from build123d import *

# Parameters (mm, degrees)
SKETCH1_R           = 3.325
SKETCH1_R_2         = 8.5
BOSS_EXTRUDE1_DEPTH = 2.5


with BuildPart() as part:
    # Sketch1 → Boss-Extrude1 (new, symmetric)
    with BuildSketch(Plane.XY):
        with BuildLine():
            ThreePointArc((60.622067271, 14.206532436), (59.125498335, 14.810906809), (57.524692071, 15.016834632))
            Line((57.524692071, 15.016834632), (56.997116089, 14.994793348))
            Line((56.997116089, 14.994793348), (37.942484943, 14.198721238))
            ThreePointArc((37.942484943, 14.198721238), (29.810784304, 16.198484397), (24.018273447, 22.245833067))
            ThreePointArc((24.018273447, 22.245833067), (11.4864831, 29.488233713), (-0.397539124, 21.225779345))
            ThreePointArc((-0.397539124, 21.225779345), (-5.665447564, 14.71634399), (-13.602008261, 12.045274491))
            Line((-13.602008261, 12.045274491), (-32.656639407, 11.249202381))
            ThreePointArc((-32.656639407, 11.249202381), (-35.431571333, 10.60798438), (-37.643867273, 8.81434161))
            ThreePointArc((-37.643867273, 8.81434161), (-38.932803958, 4.139738531), (-36.53293032, -0.073796594))
            Line((-36.53293032, -0.073796594), (10.980057512, -36.923376572))
            ThreePointArc((10.980057512, -36.923376572), (14.305396611, -37.984745832), (17.530617501, -36.649704619))
            Line((17.530617501, -36.649704619), (61.804364137, 4.034578786))
            ThreePointArc((61.804364137, 4.034578786), (63.807395856, 9.422079897), (60.622067271, 14.206532436))
        make_face()
        with Locations((14.093347289, -32.909173442)):
            Circle(SKETCH1_R, mode=Mode.SUBTRACT)
        with BuildLine():
            Line((-19.81205116, 3.778850103), (44.820399723, 6.479090855))
            ThreePointArc((44.820399723, 6.479090855), (47.71753436, 4.629103679), (46.975509685, 1.272730481))
            Line((46.975509685, 1.272730481), (15.799754589, -27.375471944))
            ThreePointArc((15.799754589, -27.375471944), (13.895096583, -28.163882109), (11.93131365, -27.537089238))
            Line((11.93131365, -27.537089238), (-21.525382137, -1.589127566))
            ThreePointArc((-21.525382137, -1.589127566), (-22.544780206, 1.693656197), (-19.81205116, 3.778850103))
        make_face(mode=Mode.SUBTRACT)
        with Locations((-32.656639407, 4.924202381)):
            Circle(SKETCH1_R, mode=Mode.SUBTRACT)
        with Locations((12.05, 16)):
            Circle(SKETCH1_R_2, mode=Mode.SUBTRACT)
        with Locations((57.524692071, 8.691834632)):
            Circle(SKETCH1_R, mode=Mode.SUBTRACT)
    extrude(amount=BOSS_EXTRUDE1_DEPTH, both=True)


solid = part.part
Model file for the job. Use its own axes, mm. Round coordinates to 2 decimals unless told otherwise and drop trailing zeros. Loops run counter-clockwise (first coordinate to the right, second up) from the corner with the lowest first, then second, coordinate; pieces in that order, holes last. Notation, with made-up numbers: (-15.5, -33) -> (37.5, -33) arc R22 ccw to (37.5, -6) -> close; hole circle Ø1 at (45, 37). An arc over 180 degrees is marked (long way). Answer as CSV lines item,"result". Start each with the question number.
1) Slice it at C-C (x = -31). List the corners of the cut face in (y, z).
2) Slice it at A-A (y = -25). List the corners of the cut face in (x, z), plus the area to 3 significant figures.
3) Probe line 1 along X through (y, z) = (9, -1.6); line 2 along Y through (x, z) = (12.05, -1.05); line 3 along X through (y, z) = (23.5, 0.25). List the from-to ranges inside material, lowest first.
4) Slice it at B-B (y = 10). List the corners of the cut face in (x, z).
5) Pin check, flat tip, straight feed: P1, Ø1, axis at y = -2, z = -1.5, coming from the +X side. Stop position of the tip, or through.
6) Slice it at D-D (z = 1.5). State how many separate pieces and enclosed holes the cut face has, plus the area to 3 significant figures.
Filled in:
1,outline,"(-4.36, -2.5) -> (2.04, -2.5) -> (2.04, 2.5) -> (-4.36, 2.5) -> close; (7.81, -2.5) -> (11.32, -2.5) -> (11.32, 2.5) -> (7.81, 2.5) -> close"
2,outline,"(-4.39, -2.5) -> (8.66, -2.5) -> (8.66, 2.5) -> (-4.39, 2.5) -> close; (18.38, -2.5) -> (30.21, -2.5) -> (30.21, 2.5) -> (18.38, 2.5) -> close"
2,area,"124 mm2"
3,line 1,"x = -37.49 to 7.23, 16.87 to 54.21, 60.84 to 63.84"
3,line 2,"y = -37.56 to -35.53, -30.29 to -27.62, 5.11 to 7.5, 24.5 to 29.5"
3,line 3,"x = 0.83 to 8.05, 16.05 to 23.27"
4,outline,"(-36.43, -2.5) -> (6.03, -2.5) -> (6.03, 2.5) -> (-36.43, 2.5) -> close; (18.07, -2.5) -> (54.47, -2.5) -> (54.47, 2.5) -> (18.07, 2.5) -> close; (60.58, -2.5) -> (63.71, -2.5) -> (63.71, 2.5) -> (60.58, 2.5) -> close"
5,P1,"stops at x = 55.78"
6,separate pieces,"1"
6,enclosed holes,"5"
6,area,"1,890 mm2"
